Verification items for the finished model (mm, model axes). A direction names the side the tool comes from. Give positions to 0.01 mm unless a question says otherwise; leave off trailing zeros. Order: outer loops, then holes, each group sorted by start corner. A loop starts at its lowest first (then second) coordinate and runs counter-clockwise, first axis right, second up. Notation, with made-up numbers: (37.25, -26) -> (88.25, -26) arc R18 ccw to (88.25, -12) -> close; hole circle Ø8 at (31, 34.5). An arc over 180 degrees is marked (long way). Return JSON: item names as keys, results as strings. Group by question number.
(1) Cross-section at C-C on z = -5. Enter the section's corners in (x, y).
(2) Release check for a two-part mould opening along X. For faces 1 (the face through (-63.196, -25, -5)), 2 (the face through (49.304, -25, -1)), 3 (the face through (-3, -53, -10)) record: pulls with the +X half, pulls with the -X half, needs draft (parallel to the pull), parting line crosses it, or undercut.
(3) Depth check by flat-ended pin: pin 1 Ø2 at (x, z) = (15, -5) entering from +Y; pin 2 Ø3.5 at (x, z) = (46.5, -1.5) entering from -Y; pin 3 Ø3.5 at (x, z) = (-27.5, -1) entering from +Y. Enter the tip coordinate at first touch or a pass-through.
(4) Cross-section at A-A on y = -34. Enter the section's corners in (x, z).
(5) Cross-section at B-B on x = 45. Enter the section's corners in (y, z), then the cut area to 3 significant figures.
(6) Cross-section at D-D on x = 20. Enter the section's corners in (y, z), then the cut area to 3 significant figures.
(7) Tool access check on faces 4 (the face through (-52, -2.9, -1)), 5 (the face through (42.304, 2, -5)), 6 (the face through (47, 0.1, -6)), 7 (the face through (-56, 5.1, -5)), 8 (the face through (-29, -55.4, -5)). Record the directions out of +Z, -Z, +X, -X, +Y, -Y that give a thin tool (end or side, any length) a straight path to the whole face; none if there is none.
(8) Thickness scan on line 1 along X through (y, z) = (-20, -3.75); line 2 along Y through (x, z) = (-50, -1.75); line 3 along X through (y, z) = (-9.5, -0.75). Record the ranges inside material, lowest first.
from build123d import *

# Parameters (mm, degrees)
F0_W     = 5
F0_H     = 20.2
F1_DEPTH = 10
F3_D     = 4.1
F3_DEPTH = 7
F3_TIP   = 1.231764269
F4_DEPTH = 3


with BuildPart() as f1:
    # F0 (on Top) → F1 (new body)
    with BuildSketch(Plane.XY):
        Polygon((-58.1956532598, -40.4000989108), (-58.1956532598, 0.0999010892), (-48.1956532598, 0.0999010892), (-48.1956532598, 5.0999010892), (-63.1956532598, 5.0999010892), (-63.1956532598, -55.4000989108), (7.1543467402, -55.4000989108), (12.1543467402, -55.4000989108), (57.3043467402, -55.4000989108), (57.3043467402, 5.0999010892), (42.3043467402, 5.0999010892), (42.3043467402, 0.0999010892), (52.3043467402, 0.0999010892), (52.3043467402, -40.4000989108), (52.3043467402, -50.4000989108), (-58.1956532598, -50.4000989108), align=None)
        with Locations((9.6543467402, -65.5000989108)):
            Rectangle(F0_W, F0_H)
    extrude(amount=-F1_DEPTH)

    # F3
    with Locations(Plane.YZ.offset(12.1543467402)):
        with Locations((-65.5000989108, -5)):
            Hole(F3_D / 2, depth=F3_DEPTH)
            with Locations((0, 0, -(F3_DEPTH + F3_TIP / 2))):  # 118° drill point
                Cone(0, F3_D / 2, F3_TIP, mode=Mode.SUBTRACT)

    # F0 (on Top) → F4 (join)
    with BuildSketch(Plane.XY):
        Polygon((-55.1956532598, -40.4000989108), (-58.1956532598, -40.4000989108), (-58.1956532598, -50.4000989108), (52.3043467402, -50.4000989108), (52.3043467402, -40.4000989108), (49.3043467402, -40.4000989108), (49.3043467402, -47.4000989108), (-55.1956532598, -47.4000989108), align=None)
        Polygon((-48.1956532598, 0.0999010892), (-58.1956532598, 0.0999010892), (-58.1956532598, -40.4000989108), (-55.1956532598, -40.4000989108), (-55.1956532598, -2.9000989108), (-48.1956532598, -2.9000989108), align=None)
        Polygon((52.3043467402, 0.0999010892), (42.3043467402, 0.0999010892), (42.3043467402, -2.9000989108), (49.3043467402, -2.9000989108), (49.3043467402, -40.4000989108), (52.3043467402, -40.4000989108), align=None)
    extrude(amount=-F4_DEPTH)


solid = f1.part
Verdict:
{
 "1": {"outline": "(-63.2, -55.4) -> (7.15, -55.4) -> (7.15, -63.45) -> (12.15, -63.45) -> (12.15, -55.4) -> (57.3, -55.4) -> (57.3, 5.1) -> (42.3, 5.1) -> (42.3, 0.1) -> (52.3, 0.1) -> (52.3, -50.4) -> (-58.2, -50.4) -> (-58.2, 0.1) -> (-48.2, 0.1) -> (-48.2, 5.1) -> (-63.2, 5.1) -> close; (7.15, -75.6) -> (12.15, -75.6) -> (12.15, -67.55) -> (7.15, -67.55) -> close"},
 "2": {"face 1": "pulls with the -X half", "face 2": "undercut", "face 3": "needs draft"},
 "3": {"pin 1": "y = -50.4", "pin 2": "y = -55.4", "pin 3": "y = -47.4"},
 "4": {"outline": "(-63.2, -10) -> (-58.2, -10) -> (-58.2, -3) -> (-55.2, -3) -> (-55.2, 0) -> (-63.2, 0) -> close; (49.3, -3) -> (52.3, -3) -> (52.3, -10) -> (57.3, -10) -> (57.3, 0) -> (49.3, 0) -> close"},
 "5": {"outline": "(-55.4, -10) -> (-50.4, -10) -> (-50.4, -3) -> (-47.4, -3) -> (-47.4, 0) -> (-55.4, 0) -> close; (-2.9, -3) -> (0.1, -3) -> (0.1, -10) -> (5.1, -10) -> (5.1, 0) -> (-2.9, 0) -> close", "area": "118 mm²"},
 "6": {"outline": "(-55.4, -10) -> (-50.4, -10) -> (-50.4, -3) -> (-47.4, -3) -> (-47.4, 0) -> (-55.4, 0) -> close", "area": "59.0 mm²"},
 "7": {"face 4": "+Z, -Z", "face 5": "+Z, -Z, +Y", "face 6": "-Z", "face 7": "+Z, -Z, +X, -X, +Y", "face 8": "+Z, -Z, -X, -Y"},
 "8": {"line 1": "-63.2 to -58.2, 52.3 to 57.3", "line 2": "-55.4 to -47.4, -2.9 to 5.1", "line 3": "-63.2 to -55.2, 49.3 to 57.3"}
}
